Part print with two shaded views. Sizes in mm from the minimum x, y, z corner. Round coordinates to 2 decimals unless told otherwise and drop trailing zeros. Order: outer loops, then holes, each group sorted by start corner. A loop starts at its lowest first (then second) coordinate and runs counter-clockwise, first axis right, second up. Notation, with made-up numbers: (61, 6) -> (108, 6) arc R36 cw to (108, 43) -> close; hole circle Ø11 at (-29, -12.5). An arc over 180 degrees is marked (long way). Answer as a JSON object with one key per item and string values.
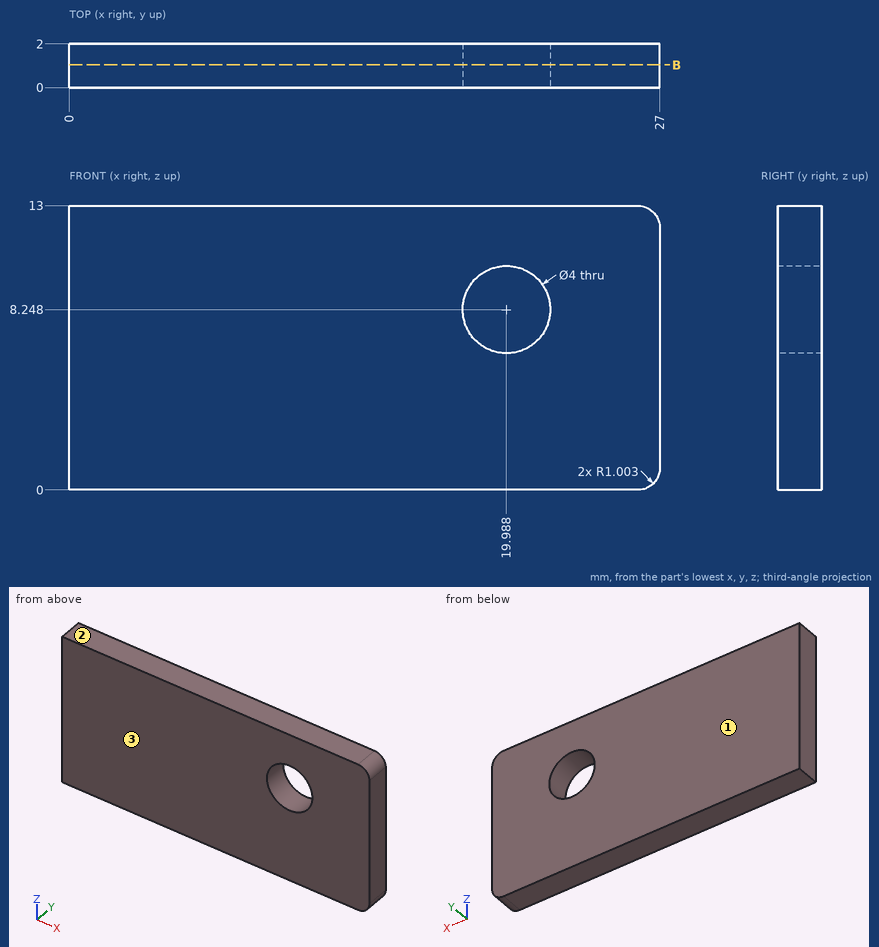
1) Cut at B-B, the plane y = 1.05. Give the cut face in (x, z), plus the area to 3 significant figures.
Checked values:
{"outline": "(0, 0) -> (26, 0) arc R1 ccw to (27, 1) -> (27, 12) arc R1 ccw to (26, 13) -> (0, 13) -> close; hole circle Ø4 at (19.99, 8.25)", "area": "338 mm²"}
2) Pull direction Y, two halves, no side cores. Call the marked faces 1, 2 and 3: pulls with the +Y half, pulls with the -Y half, needs draft (parallel to the pull), parting line crosses it, or undercut.
Checked values:
{"face 1": "pulls with the +Y half", "face 2": "needs draft", "face 3": "pulls with the -Y half"}
3) Probe L1, parallel to Z at x = 18.5, y = 1.6 (1 decimal); L2, parallel to X at y = 1.4, z = 9.25 (1 decimal); L3, parallel to Z at x = 20.75, y = 1.9. List the from-to ranges inside material, lowest first. Write a range as from..to.
Checked values:
{"L1": "z = 0..6.9, 9.6..13", "L2": "x = 0..18.3, 21.7..27", "L3": "z = 0..6.4, 10.1..13"}
